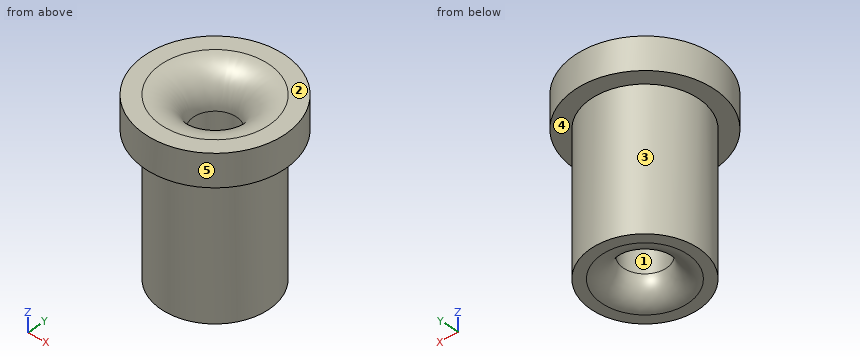
Autodesk Inventor part; units mm, degrees
ref_plane "YZ Plane" through (0, 0, 0) normal (1, 0, 0) x (0, 1, 0)
ref_plane "XZ Plane" through (0, 0, 0) normal (0, 1, 0) x (-1, 0, 0)
ref_plane "XY Plane" through (0, 0, 0) normal (0, 0, 1) x (1, 0, 0)
sketch "Sketch1" plane through (0, 0, 0) normal (0, 0, 1) x (1, 0, 0)
  line L0 (-6, 0) -> (8, 0)
  line L1 (0, 8) -> (0, -6)
  circle A0 centre (0, 0) radius 5
  dimension "d0" = 10
extrude "Extrusion1" add sketch "Sketch1" along normal blind 13
sketch "Sketch2" plane through (0, 0, 13) normal (0, 0, 1) x (1, 0, 0)
  circle A0 centre (0, 0) radius 5 construction
  circle A1 centre (0, 0) radius 6.5
  dimension "d3" = 13
extrude "Extrusion2" add sketch "Sketch2" along normal blind 3
hole "Hole1" at (0, 0, 16) direction (0, 0, -1) diameter 4 end through all
fillet "Fillet1" radius 3 1 edges at (0, 2, 16)
fillet "Fillet2" radius 2 1 edges at (0, 2, 0)
properties part number "Bushing Drill"
Can you work these out from the model? Positions are in its coordinate system, mm. Face numbers are marked on the shaded views. A direction names the side the tool comes from. Round coordinates to 2 decimals unless told otherwise and drop trailing zeros. Loops run counter-clockwise (first coordinate to the right, second up) from the corner with the lowest first, then second, coordinate; pieces in that order, holes last. Notation, with made-up numbers: (41.25, 69) - (57.25, 69) arc R24 ccw to (57.25, 86) - close; hole circle Ø5 at (-15, 58.25). An arc over 180 degrees is marked (long way). Write item = value, one per line. Start each with the question number.
(1) For P1, Ø4.5, axis at x = 0, y = 0, coming from the -Z side; P2, Ø4, axis at x = -1, z = 8.5, coming from the +Y side; P3, Ø1.5, axis at x = -2, z = 4, coming from the -Y side, each with a flat end and sliding along its axis, tell me the tip position at first contact or that it passes through.
(2) For the marked faces 4 and 5, which set-ups out of +Z, -Z, +X, -X, +Y, -Y let a thin tool reach every point of the face, with its end or its side?
(3) If we section it at C-C (z = 8.25): Please give me the cut outline in (x, y), and give its area (3 significant figures).
(4) If we mould it in two halves opening along Y, with no side actions, what happens to the marked faces 1, 2 and 3? For each: released by +Y, released by -Y, zero draft, split by the parting line, or undercut.
(5) If we section it at A-A (y = 0): Please give me the cut outline in (x, z), and give its area (3 significant figures).
(6) If I drill on probe 1 along X at (y, z) = (0, 9.75); probe 2 along Z at (x, y) = (2.75, -4), over which ranges is the centre line in solid material (lowest first)? Write a range as [from, to].
Ans:
q1.P1 = 1.03
q1.P2 = 5
q1.P3 = -4.84
q2.face_4 = -Z
q2.face_5 = +Z, -Z
q3.outline = circle Ø10 at (0, 0); hole circle Ø4 at (0, 0)
q3.area = 66.0 mm²
q4.face_1 = undercut
q4.face_2 = zero draft
q4.face_3 = split by the parting line
q5.outline = (-6.5, 13) - (-5, 13) - (-5, 0) - (-4, 0) arc R2 ccw to (-2, 2) - (-2, 13) arc R3 ccw to (-5, 16) - (-6.5, 16) - close; (2, 2) arc R2 ccw to (4, 0) - (5, 0) - (5, 13) - (6.5, 13) - (6.5, 16) - (5, 16) arc R3 ccw to (2, 13) - close
q5.area = 99.4 mm²
q6.probe_1 = [-5, -2], [2, 5]
q6.probe_2 = [0, 16]
